from build123d import *

# Parameters (mm, degrees)
SALIENTE_EXTRUIR1_DEPTH = 10
CORTAR_EXTRUIR1_DEPTH   = 8
CROQUIS3_W              = 9
CROQUIS3_H              = 2.5
SALIENTE_EXTRUIR2_DEPTH = 5
CROQUIS4_R              = 1.5499999999999994
CORTAR_EXTRUIR2_DEPTH   = 2.5
REDONDEO1_R             = 2
CROQUIS5_R              = 2.9
CORTAR_EXTRUIR3_DEPTH   = 7.6
SALIENTE_EXTRUIR3_DEPTH = 15.5
REDONDEO2_R             = 10
REDONDEO3_R             = 3
SALIENTE_EXTRUIR4_DEPTH = 5
CROQUIS8_R              = 1.5499999999999994
SALIENTE_EXTRUIR5_DEPTH = 1


with BuildPart() as part:
    # Croquis1 → Saliente-Extruir1 (new body)
    with BuildSketch(Plane(origin=(0, 0, 0), x_dir=(1, 0, 0), z_dir=(0, 1, 0))):
        Polygon((0, 0), (18.75, 0), (18.749999999999996, 16), (-3.47e-15, 16), align=None)
    extrude(amount=SALIENTE_EXTRUIR1_DEPTH)

    # Croquis2 → Cortar-Extruir1 (cut)
    with BuildSketch(Plane.XZ):
        Polygon((0, -1.7000000000000002), (18.749999999999993, -1.6999999999999997), (18.749999999999996, -14.3), (1.51e-15, -14.3), align=None)
    extrude(amount=-CORTAR_EXTRUIR1_DEPTH, mode=Mode.SUBTRACT)

    # Croquis3 → Saliente-Extruir2 (add)
    with BuildSketch(Plane.XY):
        with Locations((10.750000000000002, 1.25)):
            Rectangle(CROQUIS3_W, CROQUIS3_H)
    extrude(amount=SALIENTE_EXTRUIR2_DEPTH)

    # Croquis4 → Cortar-Extruir2 (cut)
    with BuildSketch(Plane(origin=(0, 2.5, 0), x_dir=(1, 0, 0), z_dir=(0, 1, 0))):
        with Locations(Location((10.74, -2, 0), (0, 0, 270))):
            Circle(CROQUIS4_R)
    extrude(amount=-CORTAR_EXTRUIR2_DEPTH, mode=Mode.SUBTRACT)

    # Redondeo1
    # the kernel refuses this fillet: 2 mm, written as the material it adds along each edge
    with BuildSketch(Plane(origin=(6.25, 2.5, 0), x_dir=(-1, 0, 0), z_dir=(0, -1, 0))) as redondeo1_piece_1:
        with BuildLine():
            CenterArc((REDONDEO1_R, -REDONDEO1_R), REDONDEO1_R, 90, 90)
            Line((0, -REDONDEO1_R), (0, 0))
            Line((0, 0), (REDONDEO1_R, 0))
        make_face()
    extrude(amount=2.5)
    with BuildSketch(Plane(origin=(15.25, 0, 0), x_dir=(1, 0, 0), z_dir=(0, 1, 0))) as redondeo1_piece_2:
        with BuildLine():
            CenterArc((REDONDEO1_R, -REDONDEO1_R), REDONDEO1_R, 90, 90)
            Line((0, -REDONDEO1_R), (0, 0))
            Line((0, 0), (REDONDEO1_R, 0))
        make_face()
    extrude(amount=2.5)
    with BuildSketch(Plane(origin=(15.25, 2.5, 0), x_dir=(0, 1, 0), z_dir=(-1, 0, 0))) as redondeo1_piece_3_section:
        with BuildLine():
            CenterArc((REDONDEO1_R, -REDONDEO1_R), REDONDEO1_R, 90, 90)
            Line((0, -REDONDEO1_R), (0, 0))
            Line((0, 0), (REDONDEO1_R, 0))
        make_face()
    redondeo1_piece_3 = extrude(amount=9, mode=Mode.PRIVATE)
    redondeo1_piece_3 = redondeo1_piece_3 - Plane(origin=(10.74, 2.981912580650479, 2), x_dir=(-1.8e-16, 0, 1), z_dir=(0, 1, 0)) * Cylinder(1.5499999999999994, 26, mode=Mode.PRIVATE)
    add(redondeo1_piece_3)
    with BuildSketch(Plane(origin=(6.25, 7.5, 0), x_dir=(-1, 0, 0), z_dir=(0, -1, 0))) as redondeo1_piece_4a_section:
        with BuildLine():
            CenterArc((REDONDEO1_R, -REDONDEO1_R), REDONDEO1_R, 90, 90)
            Line((0, -REDONDEO1_R), (0, 0))
            Line((0, 0), (REDONDEO1_R, 0))
        make_face()
    redondeo1_piece_4a = extrude(amount=7.5, mode=Mode.PRIVATE)
    redondeo1_piece_4a = split(redondeo1_piece_4a, bisect_by=Plane(origin=(5.797209771466349, 2.5, 0.45279022853365075), z_dir=(0, 1, 0)), keep=Keep.TOP, mode=Mode.PRIVATE)
    with BuildSketch(Plane(origin=(15.25, 2.5, 0), x_dir=(0, 1, 0), z_dir=(-1, 0, 0))) as redondeo1_piece_4b_section:
        with BuildLine():
            CenterArc((REDONDEO1_R, -REDONDEO1_R), REDONDEO1_R, 90, 90)
            Line((0, -REDONDEO1_R), (0, 0))
            Line((0, 0), (REDONDEO1_R, 0))
        make_face()
    redondeo1_piece_4b = extrude(amount=14, mode=Mode.PRIVATE)
    redondeo1_piece_4b = split(redondeo1_piece_4b, bisect_by=Plane(origin=(6.25, 2.952790228533651, 0.45279022853365075), z_dir=(-1, 0, 0)), keep=Keep.TOP, mode=Mode.PRIVATE)
    redondeo1_piece_4 = redondeo1_piece_4a & redondeo1_piece_4b
    add(redondeo1_piece_4)
    with BuildSketch(Plane(origin=(20.25, 2.5, 0), x_dir=(0, 1, 0), z_dir=(-1, 0, 0))) as redondeo1_piece_5a_section:
        with BuildLine():
            CenterArc((REDONDEO1_R, -REDONDEO1_R), REDONDEO1_R, 90, 90)
            Line((0, -REDONDEO1_R), (0, 0))
            Line((0, 0), (REDONDEO1_R, 0))
        make_face()
    redondeo1_piece_5a = extrude(amount=14, mode=Mode.PRIVATE)
    redondeo1_piece_5a = split(redondeo1_piece_5a, bisect_by=Plane(origin=(18.75, 2.952790228533651, 0.45279022853365036), z_dir=(-1, 0, 2.2e-16)), keep=Keep.TOP, mode=Mode.PRIVATE)
    redondeo1_piece_5a = split(redondeo1_piece_5a, bisect_by=Plane(origin=(15.25, 2.952790228533651, 0.45279022853365075), z_dir=(1, 0, 0)), keep=Keep.TOP, mode=Mode.PRIVATE)
    with BuildSketch(Plane(origin=(15.25, 0, 0), x_dir=(1, 0, 0), z_dir=(0, 1, 0))) as redondeo1_piece_5b_section:
        with BuildLine():
            CenterArc((REDONDEO1_R, -REDONDEO1_R), REDONDEO1_R, 90, 90)
            Line((0, -REDONDEO1_R), (0, 0))
            Line((0, 0), (REDONDEO1_R, 0))
        make_face()
    redondeo1_piece_5b = extrude(amount=7.5, mode=Mode.PRIVATE)
    redondeo1_piece_5b = split(redondeo1_piece_5b, bisect_by=Plane(origin=(15.70279022853365, 2.5, 0.45279022853364964), z_dir=(0, 1, 0)), keep=Keep.TOP, mode=Mode.PRIVATE)
    redondeo1_piece_5 = redondeo1_piece_5a & redondeo1_piece_5b
    add(redondeo1_piece_5)
    # the kernel refuses this fillet: 2 mm, written as the material it takes off along each edge
    with BuildSketch(Plane(origin=(23.749999999999996, 10, -16), x_dir=(0, -1, 0), z_dir=(-1, 0, 0))) as redondeo1_2_piece_1:
        with BuildLine():
            CenterArc((REDONDEO1_R, REDONDEO1_R), REDONDEO1_R, 180, 90)
            Line((0, REDONDEO1_R), (0, 0))
            Line((0, 0), (REDONDEO1_R, 0))
        make_face()
    extrude(amount=28.75, mode=Mode.SUBTRACT)
    with BuildSketch(Plane(origin=(6.25, 7.5, 5), x_dir=(0, 0, -1), z_dir=(0, -1, 0))) as redondeo1_2_piece_2:
        with BuildLine():
            CenterArc((REDONDEO1_R, REDONDEO1_R), REDONDEO1_R, 180, 90)
            Line((0, REDONDEO1_R), (0, 0))
            Line((0, 0), (REDONDEO1_R, 0))
        make_face()
    extrude(amount=12.5, mode=Mode.SUBTRACT)
    with BuildSketch(Plane(origin=(15.25, -5, 5), x_dir=(0, 0, -1), z_dir=(0, 1, 0))) as redondeo1_2_piece_3:
        with BuildLine():
            CenterArc((REDONDEO1_R, REDONDEO1_R), REDONDEO1_R, 180, 90)
            Line((0, REDONDEO1_R), (0, 0))
            Line((0, 0), (REDONDEO1_R, 0))
        make_face()
    extrude(amount=12.5, mode=Mode.SUBTRACT)
    with BuildSketch(Plane(origin=(-5, 10, 0), x_dir=(0, -1, 0), z_dir=(1, 0, 0))) as redondeo1_2_piece_4:
        with BuildLine():
            CenterArc((REDONDEO1_R, REDONDEO1_R), REDONDEO1_R, 180, 90)
            Line((0, REDONDEO1_R), (0, 0))
            Line((0, 0), (REDONDEO1_R, 0))
        make_face()
    extrude(amount=28.75, mode=Mode.SUBTRACT)

    # Croquis5 → Cortar-Extruir3 (cut)
    with BuildSketch(Plane(origin=(0, 10, 0), x_dir=(1, 0, 0), z_dir=(0, 1, 0))):
        with Locations(Location((10.74, -2, 0), (0, 0, 270))):
            Circle(CROQUIS5_R)
    extrude(amount=-CORTAR_EXTRUIR3_DEPTH, mode=Mode.SUBTRACT)

    # Croquis6 → Saliente-Extruir3 (add)
    with BuildSketch(Plane(origin=(0, 10, 0), x_dir=(1, 0, 0), z_dir=(0, 1, 0))):
        Polygon((-3.04e-15, 14), (3.499999999999997, 14), (3.4999999999999982, 2), (-3.04e-15, 2), align=None)
    extrude(amount=SALIENTE_EXTRUIR3_DEPTH)

    # Redondeo2
    # the kernel refuses this fillet: 10 mm, written as the material it adds along each edge
    with BuildSketch(Plane(origin=(3.499999999999997, 10, -14), x_dir=(1, 0, -1.1e-16), z_dir=(1.1e-16, 0, 1))) as redondeo2_piece_1:
        with BuildLine():
            CenterArc((REDONDEO2_R, REDONDEO2_R), REDONDEO2_R, 180, 90)
            Line((-2.22e-15, REDONDEO2_R), (0, 0))
            Line((0, 0), (REDONDEO2_R, 0))
        make_face()
    extrude(amount=12)

    # Redondeo3
    redondeo3_edges = [part.edges().sort_by_distance(p)[0] for p in [
        (1.7499999999999976, 25.5, -2),
        (1.749999999999997, 25.5, -14),
    ]]
    fillet(redondeo3_edges, radius=REDONDEO3_R)

    # Croquis7 → Saliente-Extruir4 (add)
    with BuildSketch(Plane.ZY):
        with BuildLine():
            Line((-14.3, 0), (-14.3, 8))
            Line((-14.3, 8), (-1.7000000000000002, 8))
            Line((-1.7000000000000002, 8), (-1.7000000000000002, 0))
            Line((-1.7000000000000002, 0), (0, 0))
            Line((0, 0), (0, 8))
            ThreePointArc((0, 8), (-0.5857864376269049, 9.414213562373096), (-2, 10))
            Line((-2, 10), (-2, 22.500000000000004))
            ThreePointArc((-2, 22.500000000000004), (-2.878679656440357, 24.621320343559645), (-4.999999999999999, 25.500000000000004))
            Line((-4.999999999999999, 25.500000000000004), (-11, 25.500000000000004))
            ThreePointArc((-11, 25.500000000000004), (-13.121320343559642, 24.621320343559645), (-13.999999999999998, 22.500000000000004))
            Line((-13.999999999999998, 22.500000000000004), (-14, 10))
            ThreePointArc((-14, 10), (-15.414213562373096, 9.414213562373096), (-16, 8))
            Line((-16, 8), (-16, 0))
            Line((-16, 0), (-14.3, 0))
        make_face()
    extrude(amount=SALIENTE_EXTRUIR4_DEPTH)

    # Croquis8 → Saliente-Extruir5 (add)
    # profile 1 of 2: a face of its own
    with BuildSketch(Plane.XZ):
        with BuildLine():
            Line((13.25, 5), (8.25, 5))
            ThreePointArc((8.25, 5), (6.835786437626905, 4.414213562373095), (6.25, 3.0000000000000004))
            Line((6.25, 3.0000000000000004), (6.25, 2))
            ThreePointArc((6.25, 2), (5.664213562373095, 0.5857864376269051), (4.25, 0))
            Line((4.25, 0), (-5, 1.08e-15))
            Line((-5, 1.08e-15), (-5, -1.699999999999999))
            Line((-5, -1.699999999999999), (18.749999999999993, -1.6999999999999997))
            Line((18.749999999999993, -1.6999999999999997), (18.75, 0))
            Line((18.75, 0), (17.25, 0))
            ThreePointArc((17.25, 0), (15.835786437626904, 0.5857864376269051), (15.25, 2.0000000000000004))
            Line((15.25, 2.0000000000000004), (15.25, 3))
            ThreePointArc((15.25, 3), (14.664213562373096, 4.414213562373095), (13.25, 5))
        make_face()
        with Locations(Location((10.74, 2, 0), (0, 0, 90))):
            Circle(CROQUIS8_R, mode=Mode.SUBTRACT)
    # profile 2 of 2: a face of its own
    with BuildSketch(Plane.XZ):
        Polygon((18.749999999999996, -14.3), (-5.0000000000000036, -14.299999999999999), (-5.0000000000000036, -16), (18.749999999999996, -16), align=None)
    extrude(amount=SALIENTE_EXTRUIR5_DEPTH)


solid = part.part
For this review, take the finished solid that the model builds, in its own axes (mm). A direction names the side the tool comes from. Coordinates: 2 decimals unless noted, no trailing zeros. Order: outer loops, then holes, each group sorted by start corner. A loop starts at its lowest first (then second) coordinate and runs counter-clockwise, first axis right, second up. Notation, with made-up numbers: (31, -29.5) -> (64, -29.5) arc R30 ccw to (64, -6.5) -> close; hole circle Ø1 at (-11.5, -3). An arc over 180 degrees is marked (long way). Return JSON: item names as keys, results as strings.
1. We need section B-B on x = 9.75. Write out the cut boundary in (y, z), and give its area (3 significant figures).
Answer block:
{"outline": "(-1, -16) -> (8, -16) arc R2 ccw to (10, -14) -> (10.73, -14) -> (10.73, -2) -> (10, -2) arc R2 ccw to (9.54, -0.73) -> (2.4, -0.73) -> (2.4, 0.81) -> (-1, 0.81) -> (-1, -1.7) -> (8, -1.7) -> (8, -14.3) -> (-1, -14.3) -> close; (-1, 3.19) -> (2.4, 3.19) -> (2.4, 4.73) -> (2.5, 4.73) -> (2.5, 5) -> (-1, 5) -> close", "area": "73.7 mm²"}
2. We need section D-D on y = 21.25. Write out the cut boundary in (x, z).
Answer block:
{"outline": "(-5, -14) -> (3.5, -14) -> (3.5, -2) -> (-5, -2) -> close"}
3. For pin 1 Ø10 at (x, y) = (7, 14.5) entering from -Z; pin 2 Ø5 at (x, z) = (10.74, 2) entering from +Y; pin 3 Ø9 at (x, y) = (-1.5, 3.5) entering from +Z; pin 4 Ø1 at (y, z) = (15.5, -0.5) entering from +X, all flat-tipped, find the tip position at first contact; note any pin that passes through.
Answer block:
{"pin 1": "z = -15.32", "pin 2": "y = 2.4", "pin 3": "z = 0", "pin 4": "through"}
4. We need section C-C on z = -7. Write out the cut boundary in (x, y), and give its area (3 significant figures).
Answer block:
{"outline": "(-5, 8) -> (18.75, 8) -> (18.75, 10) -> (13.5, 10) arc R10 cw to (3.5, 20) -> (3.5, 25.5) -> (-5, 25.5) -> close", "area": "201 mm²"}
5. For line 1 (Z direction, x = 10.74, y = -0.3); line 2 (Z direction, x = 10.74, y = 6.25); line 3 (Z direction, x = 1, y = 5.5), list the stretches that pass through material, from the lowest coordinate up. Write a range as from..to.
Answer block:
{"line 1": "-16..-14.3, -1.7..0.45, 3.55..5", "line 2": "-16..-14.3, -1.7..-0.9", "line 3": "-16..-14.3, -1.7..0"}
6. The part is to be moulded in two halves that separate along Z. For faces 4 (the flat face through (7, 8, -8)), 5 (the flat face through (7, -1, -15)), 6 (the cylindrical face through (6.96, 3.37, 0.35)), say which applies: +Z half, -Z half, draft (parallel to the pull), parting line (faces both ways), or undercut.
Answer block:
{"face 4": "undercut", "face 5": "draft", "face 6": "+Z half"}
7. We need section A-A on y = 3. Write out the cut boundary in (x, z), and give its area (3 significant figures).
Answer block:
{"outline": "(-5, -16) -> (18.75, -16) -> (18.75, -14.3) -> (-5, -14.3) -> close; (-5, -1.7) -> (18.75, -1.7) -> (18.75, 0) -> (17.25, 0) arc R2 cw to (15.75, 0.68) -> (13.32, 0.68) arc R2.9 cw to (8.16, 0.68) -> (5.75, 0.68) arc R2 cw to (4.25, 0) -> (-5, 0) -> close", "area": "82.3 mm²"}
8. Machinability: for faces 1 (the flat face through (9, 2.4, 3)), 2 (the flat face through (12.8, 2.5, 4.5)), 3 (the flat face through (16, 10, -8)), which of the approach directions +Z, -Z, +X, -X, +Y, -Y give a long, thin tool a straight path to every point of the face, cutting with its end or side? Answer none if there is none.
Answer block:
{"face 1": "+Y", "face 2": "+Z, +X, -X, +Y", "face 3": "+Z, -Z, +X, +Y"}
